```python
from build123d import *

# Parameters (mm, degrees)
SKETCH2_R   = 9.55
SKETCH2_R_2 = 8.05


with BuildPart() as part:
    # Sweep1: sweep along a path in Sketch1
    with BuildLine(Plane(origin=(0, 0, 0), x_dir=(1, 0, 0), z_dir=(0, 1, 0))) as sweep1_path:
        Line((250, 35), (204.142135624, 35))
        ThreePointArc((204.142135624, 35), (200.3153013, 35.761204675), (197.071067812, 37.928932188))
        Line((197.071067812, 37.928932188), (187.928932188, 47.071067812))
        ThreePointArc((187.928932188, 47.071067812), (184.6846987, 49.238795325), (180.857864376, 50))
        Line((180.857864376, 50), (30, 50))
        ThreePointArc((30, 50), (8.786796564, 41.213203436), (0, 20))
        Line((0, 20), (0, 0))
    # Sketch2 → Sweep1 (sweep)
    with BuildSketch(Plane.XY):
        Circle(SKETCH2_R)
        Circle(SKETCH2_R_2, mode=Mode.SUBTRACT)
    sweep(path=sweep1_path.line)


solid = part.part
```
Here's how the part is built. I have some questions about the finished solid (model axes, mm). A direction names the side the tool comes from. Round coordinates to 2 decimals unless told otherwise and drop trailing zeros. Order: outer loops, then holes, each group sorted by start corner. A loop starts at its lowest first (then second) coordinate and runs counter-clockwise, first axis right, second up. Notation, with made-up numbers: M 42,5.25 L 89,5.25 A15 ccw 89,10.25 Z; hole C 72.5,-24.5 d4. An arc over 180 degrees is marked long. Answer in a Markdown table with one row per item.
Item 1: If I drill on L1, parallel to Y at x = 116, z = -50; L2, parallel to X at y = -6.5, z = -33; L3, parallel to X at y = -5.75, z = -33.5, over which ranges is the centre line in solid material (lowest first)? Write a range as from..to.
A:
| item | result |
|---|---|
| L1 | y = -9.55..-8.05, 8.05..9.55 |
| L2 | x = -4.64..-2.23, 8.35..11.02, 192.11..195.57 |
| L3 | x = -5.12..-2.98, 9.72..12.16, 190.72..193.55 |
Item 2: For faces 5 (the face through (226.75, 0.42, -44.54)), 6 (the face through (104.373, 2.418, -42.322)), 7 (the face through (7.678, 2.418, -9.86)), which set-ups out of +Z, -Z, +X, -X, +Y, -Y let a thin tool reach every point of the face, with its end or its side?
A:
| item | result |
|---|---|
| face 5 | +X |
| face 6 | none |
| face 7 | +Z |
Item 3: Imagine slicing it at C-C, the plane x = 47. Write out the boundary of the cut face in (y, z).
A:
| item | result |
|---|---|
| outline | C 0,-50 d19.1; hole C 0,-50 d16.1 |
Item 4: Imagine slicing it at B-B, the plane z = -35.5. State how many separate pieces and enclosed holes the cut face has, and give its area (3 significant figures).
A:
| item | result |
|---|---|
| separate pieces | 2 |
| enclosed holes | 1 |
| area | 311 mm2 |
Item 5: Thinking about a two-plate mould opening in Z: for faces 1 (the face through (-7.58, -5.81, -9.86)), 2 (the face through (198.123, 0.354, -48.251)), 3 (the face through (-4.3, -7, 0)), 4 (the face through (104.37, 0.42, -59.54)), which applies, +Z half, -Z half, draft (parallel to the pull), parting line (faces both ways), or undercut?
A:
| item | result |
|---|---|
| face 1 | draft |
| face 2 | undercut |
| face 3 | +Z half |
| face 4 | parting line |
Item 6: I'm going to push flat-ended pins straight in: pin 1 (1 mm diameter, centred on y = -5.5, z = -46, fed in from -X); pin 2 (6 mm diameter, centred on y = -6.5, z = -27.5, fed in from -X); pin 3 (1 mm diameter, centred on x = 192.5, y = -7.5, fed in from -Z). Where does each tip first touch, or does it pass through?
A:
| item | result |
|---|---|
| pin 1 | stops at x = 1.9 |
| pin 2 | stops at x = -8.27 |
| pin 3 | stops at z = -51.83 |
Item 7: Imagine slicing it at D-D, the plane z = -4.5. Write out the boundary of the cut face in (x, y), and give its area (3 significant figures).
A:
| item | result |
|---|---|
| outline | C 0,0 d19.1; hole C 0,0 d16.1 |
| area | 82.9 mm2 |
